Check sheet for the modelled part. Datum: model origin and axes. Units: mm. Coordinates: 2 decimals unless noted, no trailing zeros. Loops run counter-clockwise (first coordinate to the right, second up) from the corner with the lowest first, then second, coordinate; pieces in that order, holes last. Notation, with made-up numbers: M 8.5,21 L 24.5,21 A24 ccw 24.5,55 Z; hole C -37,69 d9. An arc over 180 degrees is marked long. Use CSV: the item, a comma, the result in double quotes. Start each with the question number.
(1) Scan lines: line 1 (Z direction, x = 98.5, y = -6.5); line 2 (Y direction, x = 60, z = -9.6). Record each from-to range of solid material in increasing order.
(2) Section check A-A on x = 10. Record the cut outline in (y, z).
(3) Draft check along Y on faces 1 (the flat face through (79, 9, 0)), 2 (the flat face through (79, 10, 0)), 3 (the flat face through (78.9, -2.1, -9)), 4 (the cylindrical face through (12.082, -9.507, 0.273)). Enter one of: pulls with the +Y half, pulls with the -Y half, needs draft (parallel to the pull), parting line crosses it, or undercut.
(4) Section check C-C on z = 4.5. Record the cut outline in (x, y).
(5) Section check B-B on y = 0. Give the number of separate pieces and of enclosed holes in the cut face, and give its area (3 significant figures).
from build123d import *

# Parameters (mm, degrees)
SKETCH_1_W          = 20
SKETCH_1_H          = 20
EXTRUDE_1_DEPTH     = 160
SKETCH_2_R          = 2.1
CUT_EXTRUDE_1_DEPTH = 160
SKETCH_3_R          = 2.1
CUT_EXTRUDE_2_DEPTH = 162.554944214
SKETCH_4_W          = 18
SKETCH_4_H          = 18
CUT_EXTRUDE_3_DEPTH = 161.623784042


with BuildPart() as part:
    # 草图1 → 凸台-拉伸1 (new body)
    with BuildSketch(Plane(origin=(0, 0, 0), x_dir=(0, 0, -1), z_dir=(1, 0, 0))):
        Rectangle(SKETCH_1_W, SKETCH_1_H)
    extrude(amount=EXTRUDE_1_DEPTH)

    # 草图2 → 切除-拉伸1 (cut)
    with BuildSketch(Plane.XZ.offset(10)):
        with Locations(Location((10, 0, 0), (0, 0, 270))):
            Circle(SKETCH_2_R)
        with Locations(Location((30, 0, 0), (0, 0, 270))):
            Circle(SKETCH_2_R)
        with Locations(Location((50, 0, 0), (0, 0, 270))):
            Circle(SKETCH_2_R)
        with Locations(Location((110, 0, 0), (0, 0, 270))):
            Circle(SKETCH_2_R)
        with Locations(Location((130, 0, 0), (0, 0, 270))):
            Circle(SKETCH_2_R)
        with Locations(Location((150, 0, 0), (0, 0, 270))):
            Circle(SKETCH_2_R)
    extrude(amount=-CUT_EXTRUDE_1_DEPTH, mode=Mode.SUBTRACT)

    # 草图3 → 切除-拉伸2 (cut, through all)
    with BuildSketch(Plane.XY.offset(10)):
        with Locations((60, 0)):
            Circle(SKETCH_3_R)
        with Locations((80, 0)):
            Circle(SKETCH_3_R)
        with Locations((100, 0)):
            Circle(SKETCH_3_R)
    extrude(amount=-CUT_EXTRUDE_2_DEPTH, mode=Mode.SUBTRACT)

    # 草图4 → 切除-拉伸3 (cut, through all)
    with BuildSketch(Plane.ZY):
        Rectangle(SKETCH_4_W, SKETCH_4_H)
    extrude(amount=-CUT_EXTRUDE_3_DEPTH, mode=Mode.SUBTRACT)


solid = part.part
Outcome:
1,line 1,"z = -10 to -9, 9 to 10"
1,line 2,"y = -10 to -2.1, 2.1 to 10"
2,outline,"M -10,-10 L 10,-10 L 10,-2.1 L 9,-2.1 L 9,-9 L -9,-9 L -9,-2.1 L -10,-2.1 Z; M -10,2.1 L -9,2.1 L -9,9 L 9,9 L 9,2.1 L 10,2.1 L 10,10 L -10,10 Z"
3,face 1,"undercut"
3,face 2,"pulls with the +Y half"
3,face 3,"undercut"
3,face 4,"needs draft"
4,outline,"M 0,-10 L 160,-10 L 160,-9 L 0,-9 Z; M 0,9 L 160,9 L 160,10 L 0,10 Z"
5,separate pieces,"8"
5,enclosed holes,"0"
5,area,"295 mm²"
